Source: CAD feature listing. Evaluate the final solid. Frame: model axes, mm. Face numbers are marked on the shaded views. A direction names the side the tool comes from. Coordinates: 2 decimals unless noted, no trailing zeros. Order: outer loops, then holes, each group sorted by start corner. A loop starts at its lowest first (then second) coordinate and runs counter-clockwise, first axis right, second up.
Autodesk Inventor part; units mm, degrees
ref_plane "YZ Plane" through (0, 0, 0) normal (1, 0, 0) x (0, 1, 0)
ref_plane "XZ Plane" through (0, 0, 0) normal (0, 1, 0) x (-1, 0, 0)
ref_plane "XY Plane" through (0, 0, 0) normal (0, 0, 1) x (1, 0, 0)
sketch "Sketch1" plane through (0, 0, 0) normal (1, 0, 0) x (0, 1, 0)
  line L0 (-19.8, 28) -> (19.8, 28)
  line L1 (19.8, 28) -> (19.8, -28)
  line L2 (19.8, -28) -> (-19.8, -28)
  line L3 (-19.8, -28) -> (-19.8, 28)
  line L4 (-19.8, 28) -> (19.8, -28) construction
  line L5 (19.8, 28) -> (-19.8, -28) construction
  point P0 (0, 0)
  dimension "d0" = 39.6
  dimension "d1" = 56
extrude "Extrusion1" add sketch "Sketch1" along normal blind 40
sketch "Sketch2" plane through (0, -19.8, 28) normal (0, 0, 1) x (1, 0, 0)
  line L0 (7.8, 0) -> (32.2, 0)
  line L1 (32.2, 0) -> (32.2, 31.8)
  line L2 (32.2, 31.8) -> (7.8, 31.8)
  line L3 (7.8, 31.8) -> (7.8, 0)
  line L4 (0, 0) -> (40, 0)
  line L5 (40, 39.6) -> (40, 0)
  dimension "d4" = 24.4
  dimension "d5" = 31.8
  dimension "d6" = 7.8
extrude "Extrusion2" cut sketch "Sketch2" against normal blind 64
sketch "Sketch3" plane through (32.2, -19.8, 28) normal (-1, 0, 0) x (0, 0, 1)
  circle A0 centre (-12, 3.8502) radius 2.3
  circle A1 centre (-28, 3.8502) radius 2.3
  line L0 (0, 31.8) -> (0, 0)
  point P0 (-28, 19.8)
  dimension "d9" = 4.6
  dimension "d10" = 4.6
  dimension "d11" = 16
  dimension "d12" = 12
extrude "Extrusion3" add sketch "Sketch3" along normal blind 26
sketch "Sketch4" plane through (7.8, -19.8, 28) normal (1, 0, 0) x (0, 0, -1)
  line L0 (56, 0) -> (0, 0)
  line L1 (56, 0) -> (32, 0)
  line L2 (32, 0) -> (32, 8)
  line L3 (32, 8) -> (56, 8)
  line L4 (56, 8) -> (56, 0)
  point P0 (28, 19.8)
  point P1 (32, 0)
  dimension "d15" = 24
  dimension "d16" = 8
extrude "Extrusion4" add sketch "Sketch4" along normal blind 26
sketch "Sketch14" plane through (0, 19.8, 28) normal (0, 1, 0) x (1, 0, 0)
  line L0 (20, 0) -> (20, 56)
  point P0 (0, 28)
sketch "Sketch15" plane through (0, -19.8, -28) normal (0, -1, 0) x (1, 0, 0)
  line L0 (40, 0) -> (40, 56)
  line L1 (0, 0) -> (40, 0)
  line L2 (0, 56) -> (40, 56)
  line L3 (0, 0) -> (0, 56)
  point P0 (0, 28)
extrude "Extrusion7" add sketch "Sketch15" along normal blind 24
sketch "Sketch16" plane through (0, 19.8, 28) normal (0, 0, 1) x (1, 0, 0)
  line L0 (8, -47.6) -> (32, -47.6)
  line L1 (32, -47.6) -> (32, -55.6)
  line L2 (32, -55.6) -> (8, -55.6)
  line L3 (8, -55.6) -> (8, -47.6)
  line L4 (40, -63.6) -> (0, -63.6)
  line L5 (0, 0) -> (0, -63.6)
  line L6 (16, -55.6) -> (24, -55.6)
  line L7 (24, -55.6) -> (24, -63.6)
  line L8 (24, -63.6) -> (16, -63.6)
  line L9 (16, -63.6) -> (16, -55.6)
  point P0 (0, -19.8)
  dimension "d37" = 24
  dimension "d38" = 8
  dimension "d39" = 8
  dimension "d40" = 8
  dimension "d41" = 8
  dimension "d42" = 8
  dimension "d43" = 16
extrude "Extrusion8" cut sketch "Sketch16" against normal through all
chamfer "Chamfer1" distance 8 angle 45 2 edges at (40, -43.8, 0) (0, -43.8, 0)
chamfer "Chamfer2" distance 8 angle 45 2 edges at (16, -35.8, 0) (24, -35.8, 0)
split body "Split1" sketch "Sketch14" result one side removed curves L0 removed pieces at (39.5, -17.2667, 9.3333)
sketch "Sketch17" plane through (20, -27.8, -28) normal (1, 0, 0) x (0, 0, -1)
  circle A0 centre (-44, 43.6) radius 2.3
  circle A1 centre (-28, 43.6) radius 2.3
  circle A2 centre (-12, 43.6) radius 2.3
  circle A3 centre (-44, 3.6) radius 2.3
  circle A4 centre (-28, 3.6) radius 2.3
  circle A5 centre (-12, 3.6) radius 2.3
  line L0 (-56, 39.8) -> (-56, 47.6)
  line L1 (-56, 47.6) -> (0, 47.6)
  point P0 (-28, 27.8)
  dimension "d52" = 4.6
  dimension "d53" = 4.6
  dimension "d54" = 4.6
  dimension "d55" = 4.6
  dimension "d56" = 4.6
  dimension "d57" = 4.6
  dimension "d58" = 12
  dimension "d59" = 16
  dimension "d60" = 16
  dimension "d61" = 4
  dimension "d62" = 40
extrude "Extrusion9" add sketch "Sketch17" along normal blind 8
properties part number "MotorHolder_X_L"
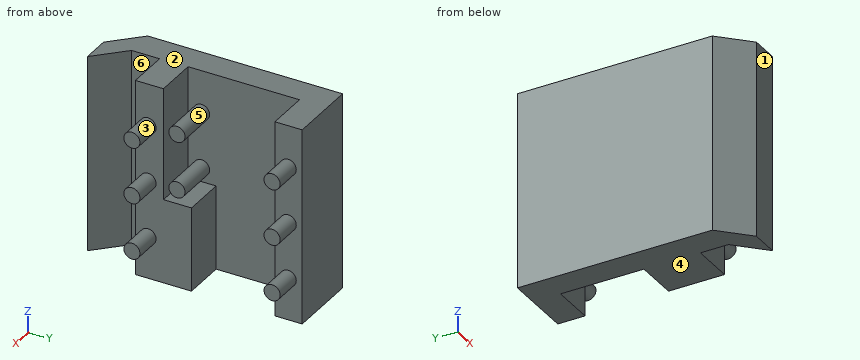
Q1. Section query C-C on y = -24.2. Output: boundary loops of the cut face in (x, z), plus the area to 3 significant figures.
Solutions:
outline: (0, -28) - (20, -28) - (20, -18.3) - (28, -18.3) - (28, -13.7) - (20, -13.7) - (20, -2.3) - (28, -2.3) - (28, 2.3) - (20, 2.3) - (20, 13.7) - (28, 13.7) - (28, 18.3) - (20, 18.3) - (20, 28) - (0, 28) - close
area: 1,230 mm2
Q2. Pull-direction query (Y, two-part tool) for the marked faces 1, 2 and 3; classes: pulls with the +Y half, pulls with the -Y half, needs draft (parallel to the pull), parting line crosses it, or undercut.
Solutions:
face 1: pulls with the -Y half
face 2: needs draft
face 3: undercut
Q3. Pin query (flat end, axial travel): P1, Ø3.5, axis at y = -15, z = -0.5, coming from the +X side; P2, Ø4, axis at y = 9.5, z = -3.5, coming from the +X side; P3, Ø6, axis at x = 25, z = -14, coming from the -Y side; P4, Ø8, axis at x = 5, z = -13, coming from the -Y side. Return the tip coordinate at first contact, or that it passes through.
Solutions:
P1: stops at x = 20
P2: stops at x = 7.8
P3: stops at y = -26.5
P4: stops at y = -43.8
Q4. Section query B-B on x = 15. Output: boundary loops of the cut face in (y, z), plus the area to 3 significant figures.
Solutions:
outline: (-43.8, -28) - (-42.8, -28) - (-42.8, 28) - (-43.8, 28) - close; (-27.8, -28) - (-11.8, -28) - (-11.8, -4) - (-19.8, -4) - (-19.8, 28) - (-27.8, 28) - close; circle Ø4.6 at (-15.95, 0); circle Ø4.6 at (-15.95, 16); (12, -28) - (19.8, -28) - (19.8, 28) - (12, 28) - close
area: 1,170 mm2
Q5. Set-up query: the marked faces 4, 5 and 6. Return all of +Z, -Z, +X, -X, +Y, -Y with unobstructed straight access to the full face (end or side cutting, diameter ignored); none if empty.
Solutions:
face 4: -Z, +X, -X, +Y, -Y
face 5: +X
face 6: +Z, -Z, +X
Q6. Section query D-D on x = 23. Output: boundary loops of the cut face in (y, z).
Solutions:
outline: circle Ø4.6 at (-24.2, -16); circle Ø4.6 at (-24.2, 0); circle Ø4.6 at (-24.2, 16); circle Ø4.6 at (15.8, -16); circle Ø4.6 at (15.8, 0); circle Ø4.6 at (15.8, 16)
Q7. Material intervals for line 1 along Y through (x, z) = (18.75, -6); line 2 along Y through (x, z) = (8.5, 8.5); line 3 along X through (y, z) = (-24.5, -8.5), sorted ascending.
Solutions:
line 1: y = -27.8 to -11.8, 12 to 19.8
line 2: y = -43.8 to -36.3, -27.8 to -19.8, 12 to 19.8
line 3: x = 0 to 20
